Drawing for the job (mm, zero at the part's lowest x, y, z). A direction names the side the tool comes from. Round coordinates to 2 decimals unless told otherwise and drop trailing zeros. Order: outer loops, then holes, each group sorted by start corner. A loop starts at its lowest first (then second) coordinate and runs counter-clockwise, first axis right, second up. Notation, with made-up numbers: M 66,24.5 L 112,24.5 A28 ccw 112,55.5 Z; hole C 25.5,42 d7. An arc over 180 degrees is marked long. One line per item, written item: value. Start each with the question number.
Item 1: Probe L1, parallel to Y at x = 6, z = 31 (3 decimals); L2, parallel to X at y = 16, z = 19.5; L3, parallel to X at y = 14, z = 19. List the from-to ranges inside material, lowest first.
Item 2: Band-saw the part on B-B, the plane z = 28.5. Write the cut outline in (x, y) (3 decimals).
Item 3: Two-plate mould, pull along Y, no slides. Class the marked faces 3, 4, 5 and 6: +Y half, -Y half, draft (parallel to the pull), parting line (faces both ways), or undercut.
Item 4: Band-saw the part on D-D, the plane z = 19.05. Write the cut outline in (x, y) (3 decimals).
Item 5: Band-saw the part on C-C, the plane x = 19.05. Write the cut outline in (y, z) (3 decimals).
Item 6: Tool access for the marked faces 1 and 2: list every direction of +Z, -Z, +X, -X, +Y, -Y with a clear straight run to the whole face (end or side of a thin tool).
Item 7: Pin check, flat tips, straight feed: pin 1 (12 mm diameter, centred on x = 28.5, y = 32, fed in from +Z) (3 decimals); pin 2 (3 mm diameter, centred on x = 27, y = 16, fed in from +Z); pin 3 (1 mm diameter, centred on x = 7, y = 24.5, fed in from +Z). Stop position of each tip, or through.
Item 8: Band-saw the part on A-A, the plane x = 28. Write the cut outline in (y, z) (3 decimals), then the cut area to 3 significant figures.
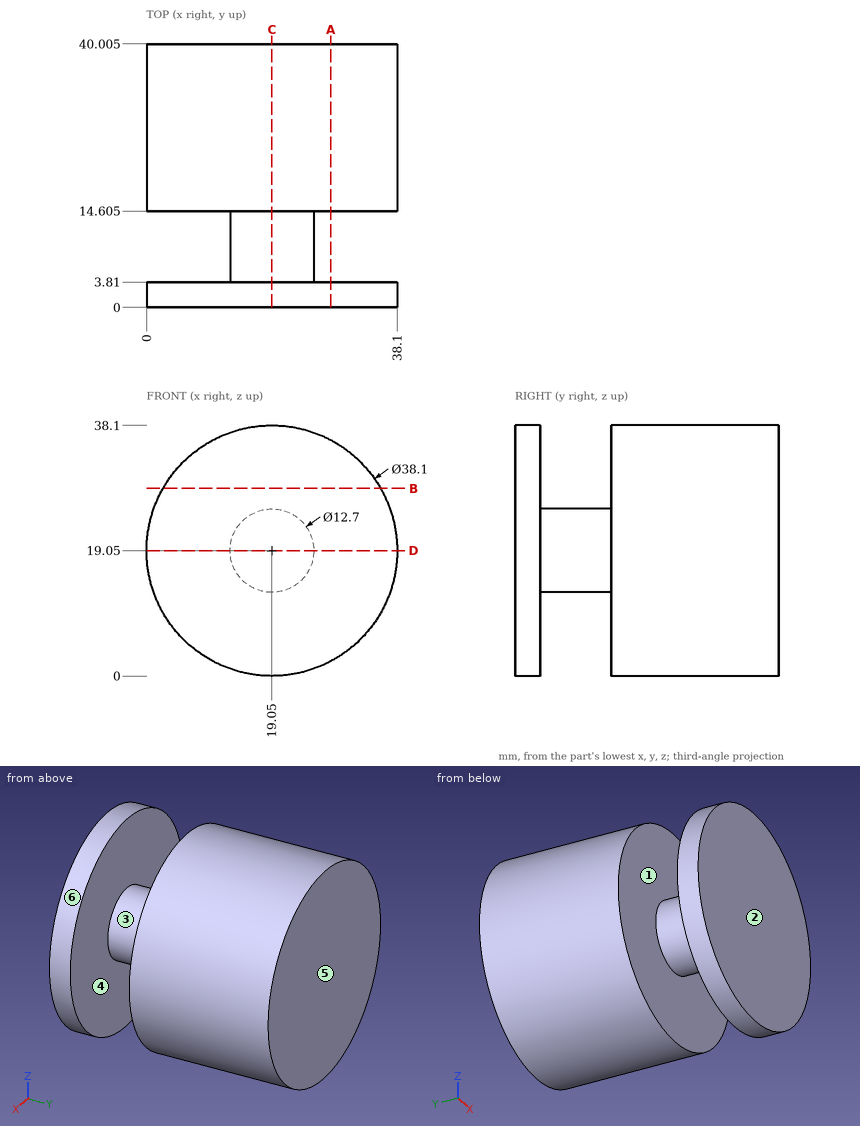
Output:
1. L1: y = 0 to 3.81, 14.605 to 40.005
1. L2: x = 0.01 to 38.09
1. L3: x = 12.7 to 25.4
2. outline: M 2.509,0 L 35.591,0 L 35.591,3.81 L 2.509,3.81 Z; M 2.509,14.605 L 35.591,14.605 L 35.591,40.005 L 2.509,40.005 Z
3. face 3: undercut
3. face 4: undercut
3. face 5: +Y half
3. face 6: draft
4. outline: M 0,0 L 38.1,0 L 38.1,3.81 L 25.4,3.81 L 25.4,14.605 L 38.1,14.605 L 38.1,40.005 L 0,40.005 L 0,14.605 L 12.7,14.605 L 12.7,3.81 L 0,3.81 Z
5. outline: M 0,0 L 3.81,0 L 3.81,12.7 L 14.605,12.7 L 14.605,0 L 40.005,0 L 40.005,38.1 L 14.605,38.1 L 14.605,25.4 L 3.81,25.4 L 3.81,38.1 L 0,38.1 Z
6. face 1: none
6. face 2: +Z, -Z, +X, -X, -Y
7. pin 1: stops at z = 37.785
7. pin 2: stops at z = 36.97
7. pin 3: stops at z = 34.2
8. outline: M 0,2.233 L 3.81,2.233 L 3.81,35.867 L 0,35.867 Z; M 14.605,2.233 L 40.005,2.233 L 40.005,35.867 L 14.605,35.867 Z
8. area: 982 mm²
